Can you work these out from the drawing? Everything is in mm from the part's minimum corner. Round coordinates to 2 decimals unless told otherwise and drop trailing zeros. Order: outer loops, then holes, each group sorted by start corner. A loop starts at its lowest first (then second) coordinate and runs counter-clockwise, first axis right, second up. Notation, with made-up numbers: (46, 49.5) - (83, 49.5) arc R18 ccw to (83, 57.5) - close; hole circle Ø6 at (-38.5, 79). An arc over 180 degrees is marked (long way). Answer as a JSON object with one key per item and string values.
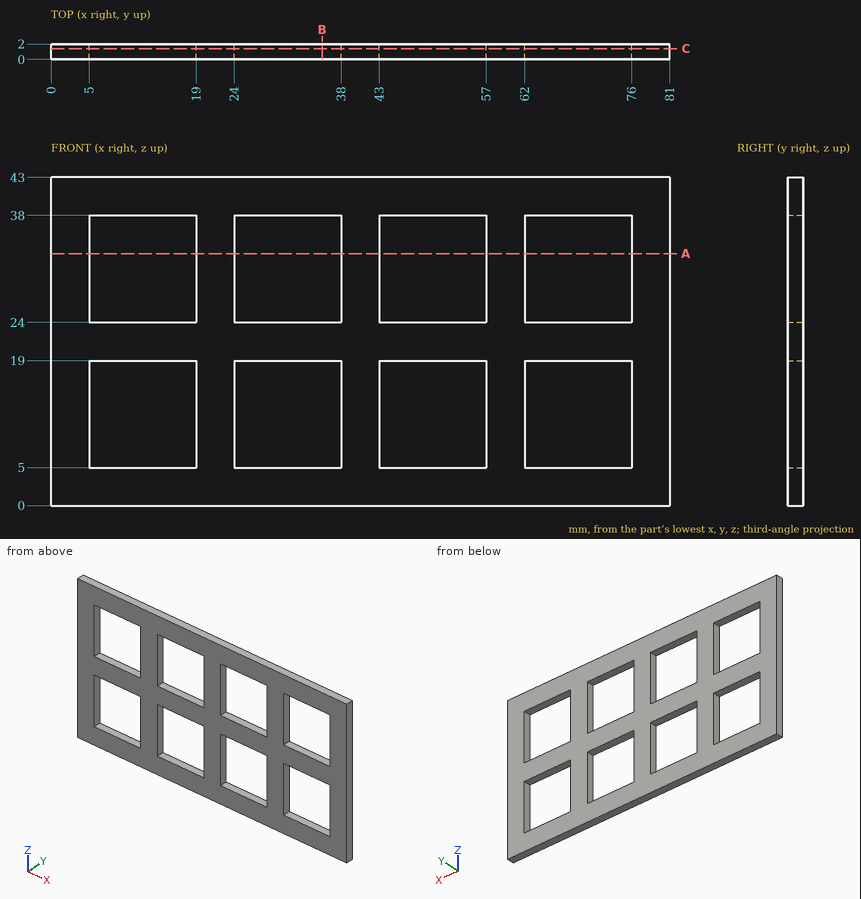
1. For P1, Ø4, axis at x = 42.5, z = 11.5, coming from the -Y side, with a flat end and sliding along its axis, tell me the tip position at first contact or that it passes through.
Responses:
{"P1": "y = 0"}
2. Imagine slicing it at B-B (x = 35.5). List the corners of the cut face in (y, z) for me, plus the area to 3 significant figures.
Responses:
{"outline": "(0, 0) - (2, 0) - (2, 5) - (0, 5) - close; (0, 19) - (2, 19) - (2, 24) - (0, 24) - close; (0, 38) - (2, 38) - (2, 43) - (0, 43) - close", "area": "30.0 mm2"}
3. If I drill on L1, parallel to X at y = 0.25, z = 15.5; L2, parallel to Z at x = 12, y = 1.6, over which ranges is the centre line in solid material (lowest first)? Write a range as [from, to].
Responses:
{"L1": "[0, 5], [19, 24], [38, 43], [57, 62], [76, 81]", "L2": "[0, 5], [19, 24], [38, 43]"}
4. Imagine slicing it at C-C (y = 1.4). Give the number of separate pieces and of enclosed holes in the cut face, plus the area to 4 significant figures.
Responses:
{"separate pieces": "1", "enclosed holes": "8", "area": "1,915 mm2"}
5. Imagine slicing it at A-A (z = 33). List the corners of the cut face in (x, y) for me, plus the area to 3 significant figures.
Responses:
{"outline": "(0, 0) - (5, 0) - (5, 2) - (0, 2) - close; (19, 0) - (24, 0) - (24, 2) - (19, 2) - close; (38, 0) - (43, 0) - (43, 2) - (38, 2) - close; (57, 0) - (62, 0) - (62, 2) - (57, 2) - close; (76, 0) - (81, 0) - (81, 2) - (76, 2) - close", "area": "50.0 mm2"}
